Study the drawing (mm; zero at the part's minimum x, y, z) and answer. A direction names the side the tool comes from. Coordinates: 2 decimals unless noted, no trailing zeros. Order: outer loops, then holes, each group sorted by start corner. A loop starts at its lowest first (then second) coordinate and runs counter-clockwise, first axis right, second up. Notation, with made-up numbers: M 76,-9 L 104,-9 A17 cw 104,20 Z; hole C -27.75,31 d7. An arc over 180 degrees is marked long. Use a Markdown table: item, result. Add a question column.
1) Find section B-B on z = 19.05. Write down the section's boundary in (x, y) (1 decimal).
2) Find section D-D on x = 215.9. Count the separate pieces of the cut face and the enclosed holes in it.
3) Find the intervals of material crossed by probe 1 along X at (y, z) = (180.34, 1.75) (1 decimal); probe 2 along Y at (x, z) = (215.9, 2.35) (1 decimal); probe 3 along Y at (x, z) = (12.7, 2) (1 decimal), in increasing order. Write a range as [from, to].
4) For the marked faces 1 and 2, determine the directions among +Z, -Z, +X, -X, +Y, -Y from which every point of the face is accessible in a straight line to the end or side of a thin tool.
5) Each of these flat-tipped pins is pushed along its axis until it touches: pin 1 Ø10 at (x, z) = (215.9, 19.05) entering from +Y (1 decimal); pin 2 Ø8.5 at (x, y) = (12.7, 53.34) entering from +Z (1 decimal). Where does it stop, or does it pass through?
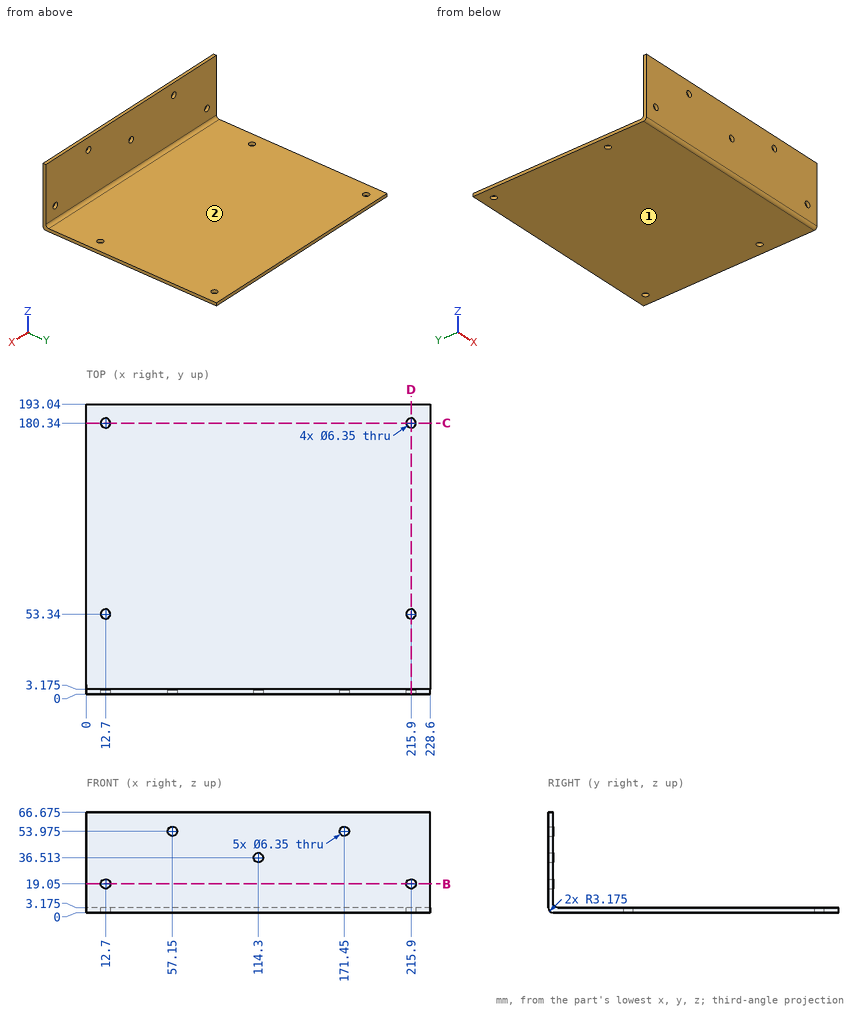
Check result:
| question | item | result |
|---|---|---|
| 1 | outline | M 0,0 L 9.5,0 L 9.5,3.2 L 0,3.2 Z; M 15.9,0 L 212.7,0 L 212.7,3.2 L 15.9,3.2 Z; M 219.1,0 L 228.6,0 L 228.6,3.2 L 219.1,3.2 Z |
| 2 | separate pieces | 4 |
| 2 | enclosed holes | 0 |
| 3 | probe 1 | x = [0, 9.5], [15.9, 212.7], [219.1, 228.6] |
| 3 | probe 2 | y = [0.1, 50.2], [56.5, 177.2], [183.5, 193] |
| 3 | probe 3 | y = [0.2, 50.2], [56.5, 177.2], [183.5, 193] |
| 4 | face 1 | -Z, +X, -X, +Y, -Y |
| 4 | face 2 | +Z, +X, -X, +Y |
| 5 | pin 1 | stops at y = 3.2 |
| 5 | pin 2 | stops at z = 3.2 |
